from build123d import *

# Parameters (mm, degrees)
BOSS_EXTRUDE2_DEPTH      = 0.79375
FILLET2_R                = 0.396875
CIRPATTERN5_COUNT        = 4
FILLET2_OF_CIRPATTERN5_R = 0.396875


with BuildPart() as part:
    # Sketch3 → Revolve2 (revolve)
    with BuildSketch(Plane(origin=(0, 0, 0), x_dir=(0, 0, -1), z_dir=(1, 0, 0)), mode=Mode.PRIVATE) as revolve2_sk:
        Polygon((95.444755644, 3.96875), (95.444755644, 0), (127, 0), (127, 3.175), (95.444755644, 7.91092396), align=None)
        with BuildLine():
            Line((0, 0.79375), (0, 0))
            Line((0, 0), (12.894755644, 0))
            ThreePointArc((12.894755644, 0), (15.684563553, 6.735192091), (22.419755644, 9.525))
            Line((22.419755644, 9.525), (79.056444567, 9.525))
            ThreePointArc((79.056444567, 9.525), (82.84913995, 8.715283085), (85.98050057, 6.427323204))
            ThreePointArc((85.98050057, 6.427323204), (88.46580805, 4.611408496), (91.476005644, 3.96875))
            Line((91.476005644, 3.96875), (95.444755644, 3.96875))
            Line((95.444755644, 3.96875), (95.444755644, 7.91092396))
            Line((95.444755644, 7.91092396), (69.85, 11.752276451))
            ThreePointArc((69.85, 11.752276451), (63.517656161, 12.462740177), (57.15, 12.7))
            Line((57.15, 12.7), (38.1, 12.7))
            ThreePointArc((38.1, 12.7), (18.1414881, 9.65411308), (0, 0.79375))
        make_face()
    revolve(revolve2_sk.sketch.rotate(Axis((0, 0, 0), (0, 0, -1)), 90), axis=Axis((0, 0, 0), (0, 0, -1)))

    # Sketch5 → Boss-Extrude2 (add, symmetric)
    with BuildSketch(Plane(origin=(0, 0, 0), x_dir=(0, 0, -1), z_dir=(1, 0, 0))):
        Polygon((120.65, 19.05), (127, 19.05), (127, 0), (88.9, 6.35), align=None)
    boss_extrude2 = extrude(amount=BOSS_EXTRUDE2_DEPTH, both=True)

    # Fillet2
    fillet2_edges = [part.edges().sort_by_distance(p)[0] for p in [
        (-0.79375, 19.05, -123.825),
        (0.79375, 19.05, -123.825),
        (-0.79375, 13.61067, -107.051675),
        (0.79375, 13.61067, -107.051675),
    ]]
    fillet(fillet2_edges, radius=FILLET2_R)

    # CirPattern5: Boss-Extrude2 ×4 about axis
    cirpattern5_axis = Axis((0, 0, 0), (0, 0, 1))
    for i in range(1, CIRPATTERN5_COUNT):
        add(boss_extrude2.rotate(cirpattern5_axis, i * 360 / CIRPATTERN5_COUNT))

    # Fillet2 of CirPattern5
    fillet2_of_cirpattern5_edges = [part.edges().sort_by_distance(p)[0] for p in [
        (-19.05, -0.79375, -123.825),
        (-19.05, 0.79375, -123.825),
        (-13.61067, -0.79375, -107.051675),
        (-13.61067, 0.79375, -107.051675),
        (0.79375, -19.05, -123.825),
        (-0.79375, -19.05, -123.825),
        (0.79375, -13.61067, -107.051675),
        (-0.79375, -13.61067, -107.051675),
        (19.05, 0.79375, -123.825),
        (19.05, -0.79375, -123.825),
        (13.61067, 0.79375, -107.051675),
        (13.61067, -0.79375, -107.051675),
    ]]
    fillet(fillet2_of_cirpattern5_edges, radius=FILLET2_OF_CIRPATTERN5_R)


solid = part.part
Read the model definition and answer for the solid it produces. Units are mm, in the model's axes. A direction names the side the tool comes from. Coordinates: 2 decimals unless noted, no trailing zeros. Loops run counter-clockwise (first coordinate to the right, second up) from the corner with the lowest first, then second, coordinate; pieces in that order, holes last. Notation, with made-up numbers: (65.25, 51.5) -> (114.25, 51.5) arc R13 ccw to (114.25, 59.5) -> close; hole circle Ø3 at (-18.75, -13.75). An arc over 180 degrees is marked (long way). Answer in a Markdown table with one row per item.
Item 1: Each of these flat-tipped pins is pushed along its axis until it touches: P1, Ø4.5, axis at y = 14.5, z = -113, coming from the +X side; P2, Ø12, axis at y = -5.5, z = -99.5, coming from the +X side; P3, Ø2.5, axis at x = 1.5, y = 0, coming from the +Z side; P4, Ø17, axis at y = -8.5, z = -116, coming from the +X side. Where does it stop, or does it pass through?
Returned:
| item | result |
|---|---|
| P1 | stops at x = 0.79 |
| P2 | stops at x = 11.92 |
| P3 | stops at z = 0 |
| P4 | stops at x = 18.4 |
Item 2: A cutting plane is placed at A-A on z = -55. Determine the outline of the cut face in (x, y) (3 decimals), plus the area to 3 significant figures.
Returned:
| item | result |
|---|---|
| outline | circle Ø25.4 at (0, 0); hole circle Ø19.05 at (0, 0) |
| area | 222 mm^2 |
Item 3: For faces 1 (the flat face through (-0.794, -11, -114)), 2 (the cylindrical face through (0.681, 13.586, -107.311)), 3 (the flat face through (0.794, 11, -114)), 4 (the flat face through (-11, 0.794, -114)), 5 (the flat face through (-0.006, -13.545, -106.888)), determine the directions among +Z, -Z, +X, -X, +Y, -Y from which every point of the face is accessible in a straight line to the end or side of a thin tool.
Returned:
| item | result |
|---|---|
| face 1 | -Z, -X, -Y |
| face 2 | +X, +Y |
| face 3 | -Z, +X, +Y |
| face 4 | -Z, -X, +Y |
| face 5 | +X, -X, -Y |
Item 4: For a pull along Z with two mould halves and no side action, classify faces 6 (the cylindrical face through (-2.06, 9.3, -51.13)), 7 (the flat face through (11, -0.794, -114)) as released by +Z, released by -Z, zero draft, split by the parting line, or undercut.
Returned:
| item | result |
|---|---|
| face 6 | undercut |
| face 7 | zero draft |
Item 5: Straight lines are drawn through the part: line 1 along Y through (x, z) = (0, -93.55); line 2 along X through (y, z) = (7, -26); line 3 along Y through (x, z) = (-7.5, -69). For each, find the intervals that lie inside material, in ascending order. Write a range as [from, to].
Returned:
| item | result |
|---|---|
| line 1 | y = [-8.21, -3.97], [3.97, 8.21] |
| line 2 | x = [-9.25, -6.46], [6.46, 9.25] |
| line 3 | y = [-9.21, -5.87], [5.87, 9.21] |
